Here's how the part is built. I have some questions about the finished solid (model axes, mm). Face numbers are marked on the shaded views. A direction names the side the tool comes from. Round coordinates to 2 decimals unless told otherwise and drop trailing zeros. Order: outer loops, then holes, each group sorted by start corner. A loop starts at its lowest first (then second) coordinate and runs counter-clockwise, first axis right, second up. Notation, with made-up numbers: (-19, 23.5) - (4, 23.5) arc R38 ccw to (4, 62.5) - close; hole circle Ø7 at (17.25, 68). An arc over 180 degrees is marked (long way). Answer as a JSON object with one key per item and string values.
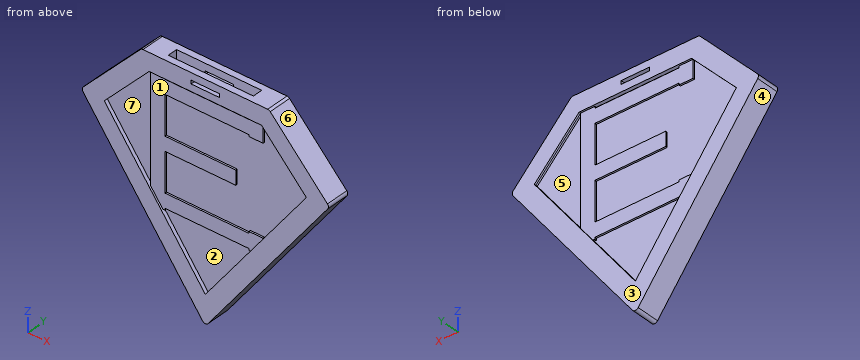
```python
from build123d import *

# Parameters (mm, degrees)
F1_DEPTH  = 3.25
F3_DEPTH  = 0.5
F5_DEPTH  = 0.5
F6_W      = 23.6895351076
F6_H      = 0.5
F7_DEPTH  = 0.5
F8_W      = 23.6895351076
F8_H      = 0.5000002682
F9_DEPTH  = 0.5
F10_W     = 24
F10_H     = 2.8
F11_DEPTH = 20
F13_DEPTH = 1.4
F14_W     = 8
F14_H     = 1
F15_DEPTH = 25
F16_R     = 1


# Not quite as in the source:
# - ends of sketch curves that miss each other by under 0.0002 mm in the source are joined


with BuildPart() as f1:
    # F0 (on Front) → F1 (new body, symmetric)
    with BuildSketch(Plane.XZ):
        Polygon((18, 18), (0, 18), (-18, 18), (-35, 0), (0, -47), (35, 0), align=None)
    extrude(amount=F1_DEPTH, both=True)

    # F2 (on face) → F3 (cut)
    with BuildSketch(Plane.XZ.offset(3.25)):
        Polygon((15.8447675538, 13), (-15.8447675538, 13), (-28.4822773709, -0.3808927475), (1.162e-07, -38.628522516), (28.4822775009, -0.3808928851), align=None)
    extrude(amount=-F3_DEPTH, mode=Mode.SUBTRACT)

    # F4 (on face) → F5 (cut)
    with BuildSketch(Plane(origin=(0, 3.25, 0), x_dir=(-1, 0, 0), z_dir=(0, 1, 0))):
        Polygon((28.482277527, -0.3808925379), (15.8447676545, 13.0000002682), (-15.8447670441, 13.0000002682), (-28.4822772579, -0.3808928993), (0, -38.6285223599), align=None)
    extrude(amount=-F5_DEPTH, mode=Mode.SUBTRACT)

    # F6 (on face) → F7 (cut)
    with BuildSketch(Plane.XZ.offset(2.75)):
        Polygon((-15.8447675538, -17.3512630734), (-15.8447675538, 13), (-28.4822773709, -0.3808927475), align=None)
        Polygon((28.4822775009, -0.3808928851), (15.8447675538, 13), (15.8447675538, 8), (11.8447675538, 8), (11.8447675538, 8.5), (-11.8447675538, 8.5), (-11.8447675538, -2.5), (8.1552324462, -2.5), (8.1552324462, -6.5), (-11.8447675538, -6.5), (-11.8447675538, -17.5), (11.8447675538, -17.5), (11.8447675538, -17), (15.8447675538, -17), (15.8447675538, -17.3512633855), align=None)
        with Locations((0, 12.75)):
            Rectangle(F6_W, F6_H)
        Polygon((-11.8447675538, -22), (-12.3829421829, -22), (1.162e-07, -38.628522516), (12.3829424153, -22), (11.8447675538, -22), (11.8447675538, -21.5), (-11.8447675538, -21.5), align=None)
    extrude(amount=-F7_DEPTH, mode=Mode.SUBTRACT)

    # F8 (on face) → F9 (cut)
    with BuildSketch(Plane(origin=(0, 2.75, 0), x_dir=(-1, 0, 0), z_dir=(0, 1, 0))):
        Polygon((-11.8447675538, -2.5), (8.1552324462, -2.5), (8.1552324462, -6.5), (-11.8447675538, -6.5), (-11.8447675538, -17.5), (11.8447675538, -17.5), (11.8447675538, -17), (15.8447675538, -17), (15.8447675538, -17.3512630734), (28.482277527, -0.3808925379), (15.8447676545, 13.0000002682), (15.8447675538, 8), (11.8447675538, 8), (11.8447675538, 8.5), (-11.8447675538, 8.5), align=None)
        Polygon((11.8447675538, -21.5), (-11.8447675538, -21.5), (-11.8447675538, -22), (-12.3829424153, -22), (0, -38.6285223599), (12.3829421829, -22), (11.8447675538, -22), align=None)
        Polygon((-15.8447675538, -17.3512630734), (-15.8447675538, 13), (-28.4822772579, -0.3808928993), align=None)
        with Locations((0, 12.7500001341)):
            Rectangle(F8_W, F8_H)
    extrude(amount=-F9_DEPTH, mode=Mode.SUBTRACT)

    # F10 (on face) → F11 (cut)
    with BuildSketch(Plane.XY.offset(18)):
        Rectangle(F10_W, F10_H)
    extrude(amount=-F11_DEPTH, mode=Mode.SUBTRACT)

    # F12 (on Front) → F13 (cut, symmetric)
    with BuildSketch(Plane.XZ):
        with BuildLine():
            Line((12, -2), (-12, -2))
            ThreePointArc((-12, -2), (0, -14), (12, -2))
        make_face()
    extrude(amount=F13_DEPTH, both=True, mode=Mode.SUBTRACT)

    # F14 (on face) → F15 (cut)
    with BuildSketch(Plane.XZ.offset(3.25)):
        with Locations((0, 15.5)):
            Rectangle(F14_W, F14_H)
    extrude(amount=-F15_DEPTH, mode=Mode.SUBTRACT)

    # F16
    f16_edges = [f1.edges().sort_by_distance(p)[0] for p in [
        (0, 0, -47),
        (35, 0, 0),
        (-35, 0, 0),
        (-18, 0, 18),
        (18, 0, 18),
    ]]
    fillet(f16_edges, radius=F16_R)


solid = f1.part
```
1. Imagine slicing it at C-C (z = -27). List the corners of the cut face in (x, y) for me.
Responses:
{"outline": "(-14.89, -3.25) - (-8.66, -3.25) - (-8.66, -2.25) - (8.66, -2.25) - (8.66, -3.25) - (14.89, -3.25) - (14.89, 3.25) - (8.66, 3.25) - (8.66, 2.25) - (-8.66, 2.25) - (-8.66, 3.25) - (-14.89, 3.25) - close"}
2. If I drill on L1, parallel to Z at x = 0, y = 2; L2, parallel to Y at x = -18.5, z = 1; L3, parallel to Y at x = -0.5, z = -18, over which ranges is the centre line in solid material (lowest first)? Write a range as [from, to].
Responses:
{"L1": "[-46.33, 15], [16, 18]", "L2": "[-2.25, 2.25]", "L3": "[-2.75, 2.75]"}
3. Thinking about a two-plate mould opening in X: for the marked faces 1, 2, 3 and 4, which applies, pulls with the +X half, pulls with the -X half, needs draft (parallel to the pull), parting line crosses it, or undercut?
Responses:
{"face 1": "undercut", "face 2": "undercut", "face 3": "needs draft", "face 4": "pulls with the -X half"}
4. For P1, Ø0.6, axis at x = 0.5, y = -2.5, coming from the -Z side; P2, Ø1.4, axis at y = 0, z = 5, coming from the -X side; P3, Ø12, axis at x = 1, z = -27, coming from the +Y side, each with a flat end and sliding along its axis, tell me the tip position at first contact or that it passes through.
Responses:
{"P1": "z = -46.31", "P2": "x = -30.94", "P3": "y = 2.75"}
5. Imagine slicing it at B-B (z = 6.5). List the corners of the cut face in (x, y) for me.
Responses:
{"outline": "(-28.86, -3.25) - (-21.98, -3.25) - (-21.98, -2.25) - (-15.84, -2.25) - (-15.84, -2.75) - (-11.84, -2.75) - (-11.84, -2.25) - (21.98, -2.25) - (21.98, -3.25) - (28.86, -3.25) - (28.86, 3.25) - (21.98, 3.25) - (21.98, 2.25) - (15.84, 2.25) - (15.84, 2.75) - (11.84, 2.75) - (11.84, 2.25) - (-21.98, 2.25) - (-21.98, 3.25) - (-28.86, 3.25) - close; hole (-12, -1.4) - (12, -1.4) - (12, 1.4) - (-12, 1.4) - close"}
6. For the marked faces 5, 6 and 7, which set-ups out of +Z, -Z, +X, -X, +Y, -Y let a thin tool reach every point of the face, with its end or its side?
Responses:
{"face 5": "+Y", "face 6": "+Z, +X, +Y, -Y", "face 7": "-Y"}
7. Imagine slicing it at D-D (z = -11). List the corners of the cut face in (x, y) for me.
Responses:
{"outline": "(-26.81, -3.25) - (-20.57, -3.25) - (-20.57, -2.25) - (-15.84, -2.25) - (-15.84, -2.75) - (-11.84, -2.75) - (-11.84, -2.25) - (20.57, -2.25) - (20.57, -3.25) - (26.81, -3.25) - (26.81, 3.25) - (20.57, 3.25) - (20.57, 2.25) - (15.84, 2.25) - (15.84, 2.75) - (11.84, 2.75) - (11.84, 2.25) - (-20.57, 2.25) - (-20.57, 3.25) - (-26.81, 3.25) - close; hole (-7.94, -1.4) - (7.94, -1.4) - (7.94, 1.4) - (-7.94, 1.4) - close"}
8. Imagine slicing it at A-A (y = 0.5). List the corners of the cut face in (x, z) for me.
Responses:
{"outline": "(-34.5, -0.67) - (-0.8, -45.92) arc R1 ccw to (0.8, -45.92) - (34.5, -0.67) arc R1 ccw to (34.42, 0.61) - (18.3, 17.69) arc R1 ccw to (17.57, 18) - (12, 18) - (12, -2) arc R12 cw to (-12, -2) - (-12, 18) - (-17.57, 18) arc R1 ccw to (-18.3, 17.69) - (-34.42, 0.61) arc R1 ccw to start"}
